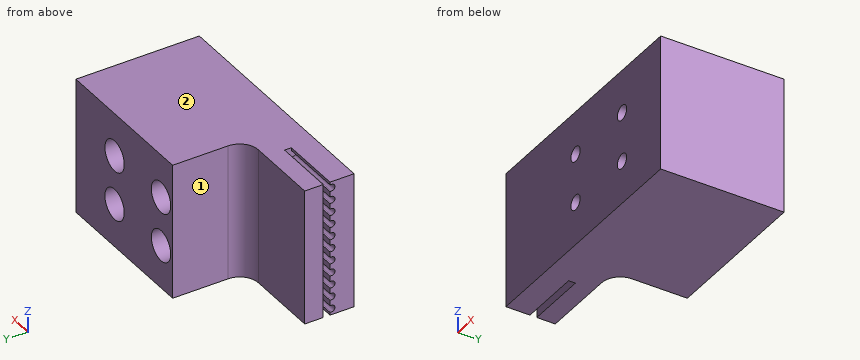
```python
from build123d import *

# Parameters (mm, degrees)
SKETCH_1_W                   = 20
SKETCH_1_H                   = 30
EXTRUDE_1_DEPTH              = 30
CUT_EXTRUDE_1_DEPTH          = 10
SKETCH_15_W                  = 20
SKETCH_15_H                  = 30
CUT_EXTRUDE_6_DEPTH          = 10
SKETCH_16_W                  = 30
SKETCH_16_H                  = 20
EXTRUDE_5_DEPTH              = 20
HOLE_WIZARD_M2_2_D           = 2.4
HOLE_WIZARD_M2_2_CSINK_D     = 2.45
HOLE_WIZARD_M2_2_CSINK_ANGLE = 90
SKETCH_20_R                  = 2.5
CUT_EXTRUDE_7_DEPTH          = 12
SKETCH_21_W                  = 15
SKETCH_21_H                  = 12
CUT_EXTRUDE_8_DEPTH          = 31
SKETCH_22_W                  = 40
SKETCH_22_H                  = 4
CUT_EXTRUDE_9_DEPTH          = 21
FILLET_1_R                   = 3


with BuildPart() as part:
    # 草图1 → 凸台-拉伸1 (new body)
    with BuildSketch(Plane.XY):
        with Locations((10, 15)):
            Rectangle(SKETCH_1_W, SKETCH_1_H)
    extrude(amount=EXTRUDE_1_DEPTH)

    # 草图3 → 切除-拉伸1 (cut)
    with BuildSketch(Plane.ZY):
        with BuildLine():
            Line((11.550000034, 3.65), (11.550000034, 3.899807334))
            Line((11.550000034, 3.899807334), (12.450000034, 3.899807334))
            Line((12.450000034, 3.899807334), (12.450000034, 3.649807334))
            ThreePointArc((12.450000034, 3.649807334), (13, 3.1), (13.549999966, 3.649807334))
            Line((13.549999966, 3.649807334), (13.549999966, 3.899807334))
            Line((13.549999966, 3.899807334), (14.449999966, 3.899807334))
            Line((14.449999966, 3.899807334), (14.449999966, 3.65))
            ThreePointArc((14.449999966, 3.65), (15, 3.099999966), (15.550000034, 3.65))
            Line((15.550000034, 3.65), (15.550000034, 3.899807334))
            Line((15.550000034, 3.899807334), (16.450000034, 3.899807334))
            Line((16.450000034, 3.899807334), (16.450000034, 3.649807334))
            ThreePointArc((16.450000034, 3.649807334), (17, 3.1), (17.549999966, 3.649807334))
            Line((17.549999966, 3.649807334), (17.549999966, 3.899807334))
            Line((17.549999966, 3.899807334), (18.449999966, 3.899807334))
            Line((18.449999966, 3.899807334), (18.449999966, 3.65))
            ThreePointArc((18.449999966, 3.65), (19, 3.099999966), (19.550000034, 3.65))
            Line((19.550000034, 3.65), (19.550000034, 3.899807334))
            Line((19.550000034, 3.899807334), (20.450000034, 3.899807334))
            Line((20.450000034, 3.899807334), (20.450000034, 3.649807334))
            ThreePointArc((20.450000034, 3.649807334), (21, 3.1), (21.549999966, 3.649807334))
            Line((21.549999966, 3.649807334), (21.549999966, 3.899807334))
            Line((21.549999966, 3.899807334), (22.449999966, 3.899807334))
            Line((22.449999966, 3.899807334), (22.449999966, 3.65))
            ThreePointArc((22.449999966, 3.65), (23, 3.099999966), (23.550000034, 3.65))
            Line((23.550000034, 3.65), (23.550000034, 3.899807334))
            Line((23.550000034, 3.899807334), (24.450000034, 3.899807334))
            Line((24.450000034, 3.899807334), (24.450000034, 3.649807334))
            ThreePointArc((24.450000034, 3.649807334), (25, 3.1), (25.549999966, 3.649807334))
            Line((25.549999966, 3.649807334), (25.549999966, 3.899807334))
            Line((25.549999966, 3.899807334), (26.449999966, 3.899807334))
            Line((26.449999966, 3.899807334), (26.449999966, 3.65))
            ThreePointArc((26.449999966, 3.65), (27, 3.099999966), (27.550000034, 3.65))
            Line((27.550000034, 3.65), (27.550000034, 3.899807334))
            Line((27.550000034, 3.899807334), (28.450000034, 3.899807334))
            Line((28.450000034, 3.899807334), (28.450000034, 3.649807334))
            ThreePointArc((28.450000034, 3.649807334), (29, 3.1), (29.549999966, 3.649807334))
            Line((29.549999966, 3.649807334), (29.549999966, 3.899807334))
            Line((29.549999966, 3.899807334), (30.449999966, 3.899807334))
            Line((30.449999966, 3.899807334), (30.449999966, 3.65))
            ThreePointArc((30.449999966, 3.65), (30.61109127, 3.26109127), (31, 3.1))
            Line((31, 3.1), (31, 5))
            Line((31, 5), (15, 5))
            Line((15, 5), (-1, 5))
            Line((-1, 5), (-1, 3.1))
            ThreePointArc((-1, 3.1), (-0.61109127, 3.26109127), (-0.449999966, 3.65))
            Line((-0.449999966, 3.65), (-0.449999966, 3.899807334))
            Line((-0.449999966, 3.899807334), (0.450000034, 3.899807334))
            Line((0.450000034, 3.899807334), (0.450000034, 3.649807334))
            ThreePointArc((0.450000034, 3.649807334), (1, 3.1), (1.549999966, 3.649807334))
            Line((1.549999966, 3.649807334), (1.549999966, 3.899807334))
            Line((1.549999966, 3.899807334), (2.449999966, 3.899807334))
            Line((2.449999966, 3.899807334), (2.449999966, 3.65))
            ThreePointArc((2.449999966, 3.65), (3, 3.099999966), (3.550000034, 3.65))
            Line((3.550000034, 3.65), (3.550000034, 3.899807334))
            Line((3.550000034, 3.899807334), (4.450000034, 3.899807334))
            Line((4.450000034, 3.899807334), (4.450000034, 3.649807334))
            ThreePointArc((4.450000034, 3.649807334), (5, 3.1), (5.549999966, 3.649807334))
            Line((5.549999966, 3.649807334), (5.549999966, 3.899807334))
            Line((5.549999966, 3.899807334), (6.449999966, 3.899807334))
            Line((6.449999966, 3.899807334), (6.449999966, 3.65))
            ThreePointArc((6.449999966, 3.65), (7, 3.099999966), (7.550000034, 3.65))
            Line((7.550000034, 3.65), (7.550000034, 3.899807334))
            Line((7.550000034, 3.899807334), (8.450000034, 3.899807334))
            Line((8.450000034, 3.899807334), (8.450000034, 3.649807334))
            ThreePointArc((8.450000034, 3.649807334), (9, 3.1), (9.549999966, 3.649807334))
            Line((9.549999966, 3.649807334), (9.549999966, 3.899807334))
            Line((9.549999966, 3.899807334), (10.449999966, 3.899807334))
            Line((10.449999966, 3.899807334), (10.449999966, 3.65))
            ThreePointArc((10.449999966, 3.65), (11, 3.099999966), (11.550000034, 3.65))
        make_face()
    extrude(amount=-CUT_EXTRUDE_1_DEPTH, mode=Mode.SUBTRACT)

    # 草图15 → 切除-拉伸6 (cut)
    with BuildSketch(Plane(origin=(0, 30, 0), x_dir=(1, 0, 0), z_dir=(0, 1, 0))):
        with Locations((10, -15)):
            Rectangle(SKETCH_15_W, SKETCH_15_H)
    extrude(amount=-CUT_EXTRUDE_6_DEPTH, mode=Mode.SUBTRACT)

    # 草图16 → 凸台-拉伸5 (add)
    with BuildSketch(Plane(origin=(20, 0, 0), x_dir=(0, 0, -1), z_dir=(1, 0, 0))):
        with Locations((-15, 10)):
            Rectangle(SKETCH_16_W, SKETCH_16_H)
    extrude(amount=EXTRUDE_5_DEPTH)

    # M2 间隙孔2 (through all)
    with Locations(Plane(origin=(0, 20, 0), x_dir=(1, 0, 0), z_dir=(0, 1, 0))):
        with Locations((18, -19), (18, -11), (30, -11), (30, -19)):
            CounterSinkHole(HOLE_WIZARD_M2_2_D / 2, HOLE_WIZARD_M2_2_CSINK_D / 2, counter_sink_angle=HOLE_WIZARD_M2_2_CSINK_ANGLE)

    # 草图20 → 切除-拉伸7 (cut)
    with BuildSketch(Plane(origin=(0, 20, 0), x_dir=(1, 0, 0), z_dir=(0, 1, 0))):
        with Locations((18, -11)):
            Circle(SKETCH_20_R)
        with Locations((30, -11)):
            Circle(SKETCH_20_R)
        with Locations((30, -19)):
            Circle(SKETCH_20_R)
        with Locations((18, -19)):
            Circle(SKETCH_20_R)
    extrude(amount=-CUT_EXTRUDE_7_DEPTH, mode=Mode.SUBTRACT)

    # 草图21 → 切除-拉伸8 (cut, through all)
    with BuildSketch(Plane(origin=(0, 0, 0), x_dir=(-1, 0, 0), z_dir=(0, 0, -1))):
        with Locations((-7.5, 14)):
            Rectangle(SKETCH_21_W, SKETCH_21_H)
    extrude(amount=-CUT_EXTRUDE_8_DEPTH, mode=Mode.SUBTRACT)

    # 草图22 → 切除-拉伸9 (cut, through all)
    with BuildSketch(Plane.XZ):
        with Locations((20, 28)):
            Rectangle(SKETCH_22_W, SKETCH_22_H)
        with Locations((20, 2)):
            Rectangle(SKETCH_22_W, SKETCH_22_H)
    extrude(amount=-CUT_EXTRUDE_9_DEPTH, mode=Mode.SUBTRACT)

    # 圆角1
    fillet_1_edges = [part.edges().sort_by_distance(p)[0] for p in [
        (15, 8, 15),
    ]]
    fillet(fillet_1_edges, radius=FILLET_1_R)


solid = part.part
```
Here's how the part is built. I have some questions about the finished solid (model axes, mm). Face numbers are marked on the shaded views. A direction names the side the tool comes from. Give positions to 0.01 mm unless a question says otherwise; leave off trailing zeros. Loops run counter-clockwise (first coordinate to the right, second up) from the corner with the lowest first, then second, coordinate; pieces in that order, holes last. Notation, with made-up numbers: M -20,-28 L -7,-28 A26 cw -7,-12 Z; hole C 47,70 d9. An arc over 180 degrees is marked long. Return JSON: item names as keys, results as strings.
Item 1: Please list where these lines run through material, in increasing order: line 1 (X direction, y = 4.5, z = 19); line 2 (Z direction, x = 30, y = 3.75); line 3 (X direction, y = 15.5, z = 19).
A:
{"line 1": "x = 10 to 16.8, 19.2 to 28.8, 31.2 to 40", "line 2": "z = 4 to 9.8, 12.2 to 17.8, 20.2 to 26", "line 3": "x = 15 to 15.5, 20.5 to 27.5, 32.5 to 40"}
Item 2: Imagine slicing it at C-C on z = 11. List the corners of the cut face in (x, y) for me, then the cut area to 3 significant figures.
A:
{"outline": "M 0,0 L 16.8,0 L 16.8,8 L 15.5,8 L 15.5,20 L 15,20 L 15,11 A3 cw 12,8 L 0,8 L 0,5 L 10,5 L 10,3.1 L 0,3.1 Z; M 19.2,0 L 28.8,0 L 28.8,8 L 27.5,8 L 27.5,20 L 20.5,20 L 20.5,8 L 19.2,8 Z; M 31.2,0 L 40,0 L 40,20 L 32.5,20 L 32.5,8 L 31.2,8 Z", "area": "445 mm^2"}
Item 3: I'm going to push flat-ended pins straight in: pin 1 Ø1 at (x, z) = (5, 8) entering from +Y; pin 2 Ø2.5 at (y, z) = (16, 11) entering from -X. Where does each tip first touch, or does it pass through?
A:
{"pin 1": "stops at y = 8", "pin 2": "stops at x = 15"}
Item 4: Imagine slicing it at A-A on y = 18.25. List the corners of the cut face in (x, z) for me.
A:
{"outline": "M 15,4 L 40,4 L 40,26 L 15,26 Z; hole C 18,11 d5; hole C 18,19 d5; hole C 30,11 d5; hole C 30,19 d5"}
Item 5: On a 3-axis mill with a long thin cutter (end or side, diameter ignored), from which of +Z, -Z, +X, -X, +Y, -Y can I reach the whole of each face in a straight line? I mean the marked faces 1 and 2. Say none if no direction works.
A:
{"face 1": "+Z, -Z, -X, +Y", "face 2": "+Z, +X, -X, +Y, -Y"}
Item 6: Imagine slicing it at D-D on z = 25. List the corners of the cut face in (x, y) for me, then the cut area to 3 significant figures.
A:
{"outline": "M 0,0 L 40,0 L 40,20 L 15,20 L 15,11 A3 cw 12,8 L 0,8 L 0,5 L 10,5 L 10,3.1 L 0,3.1 Z", "area": "603 mm^2"}
Item 7: Imagine slicing it at B-B on x = 30. List the corners of the cut face in (y, z) for me, then the cut area to 3 significant figures.
A:
{"outline": "M 0,4 L 20,4 L 20,8.5 L 8,8.5 L 8,9.8 L 0,9.8 Z; M 0,12.2 L 8,12.2 L 8,13.5 L 20,13.5 L 20,16.5 L 8,16.5 L 8,17.8 L 0,17.8 Z; M 0,20.2 L 8,20.2 L 8,21.5 L 20,21.5 L 20,26 L 0,26 Z", "area": "282 mm^2"}
